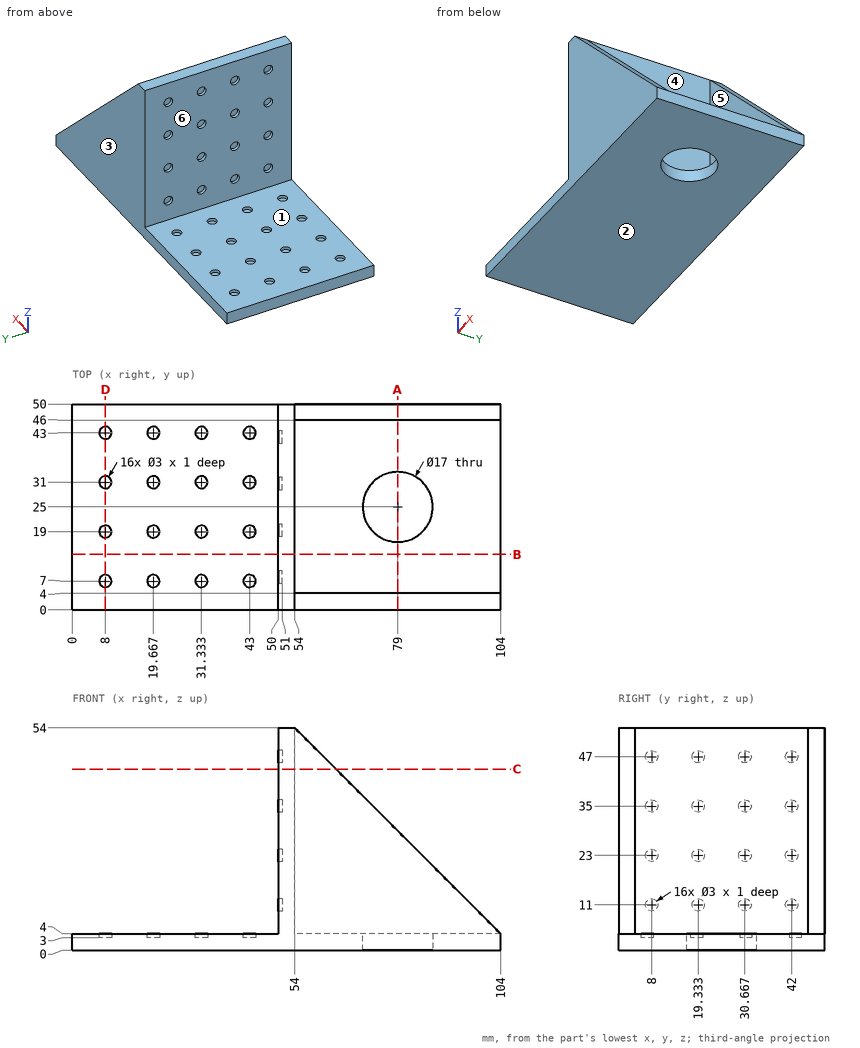
Verification items for this drawing (mm, ordinates from the low corner). A direction names the side the tool comes from. Give positions to 0.01 mm unless a question says otherwise; leave off trailing zeros. Loops run counter-clockwise (first coordinate to the right, second up) from the corner with the lowest first, then second, coordinate; pieces in that order, holes last. Notation, with made-up numbers: M 12,-6.5 L 48,-6.5 A34 ccw 48,29.5 Z; hole C -19.75,16 d4. An arc over 180 degrees is marked long. Answer as a JSON object with one key per item and string values. Group by question number.
Item 1: Sectioned sample at C-C on z = 44. Record the boundary of the cut face in (x, y), plus the area to 3 significant figures.
Item 2: Sectioned sample at D-D on x = 8. Record the boundary of the cut face in (y, z), plus the area to 3 significant figures.
Item 3: Gauge pin test, flat ends, axial feed: pin 1 (3.5 mm diameter, centred on y = 19.33, z = 47, fed in from +X); pin 2 (12 mm diameter, centred on y = 24, z = 23, fed in from -X); pin 3 (4 mm diameter, centred on x = 32.5, y = 28.5, fed in from +Z). Record the tip position at first contact, or that the pin passes through.
Item 4: Access from +Z, -Z, +X, -X, +Y, -Y to the whole of each face (thin tool, end or side, straight path). Record for the marked faces 1 and 2.
Item 5: Sectioned sample at B-B on y = 13.5. Record the boundary of the cut face in (x, z), plus the area to 3 significant figures.
Item 6: Material ranges on L1, parallel to Y at x = 59, z = 39; L2, parallel to Z at x = 34.5, y = 30; L3, parallel to X at y = 28, z = 33, recorded low to high.
Item 7: Mould release check, pull along Y, two halves, no side actions. Record for the marked faces 3, 4, 5 and 6: pulls with the +Y half, pulls with the -Y half, needs draft (parallel to the pull), parting line crosses it, or undercut.
Item 8: Sectioned sample at A-A on x = 79. Record the boundary of the cut face in (y, z), plus the area to 3 significant figures.
Findings below:
{
 "1": {"outline": "M 50,0 L 64,0 L 64,4 L 54,4 L 54,46 L 64,46 L 64,50 L 50,50 Z", "area": "280 mm2"},
 "2": {"outline": "M 0,0 L 50,0 L 50,4 L 44.5,4 L 44.5,3 L 41.5,3 L 41.5,4 L 32.5,4 L 32.5,3 L 29.5,3 L 29.5,4 L 20.5,4 L 20.5,3 L 17.5,3 L 17.5,4 L 8.5,4 L 8.5,3 L 5.5,3 L 5.5,4 L 0,4 Z", "area": "188 mm2"},
 "3": {"pin 1": "x = 54", "pin 2": "x = 50", "pin 3": "z = 4"},
 "4": {"face 1": "+Z, -X, +Y, -Y", "face 2": "-Z, +X, -X, +Y, -Y"},
 "5": {"outline": "M 0,0 L 104,0 L 104,4 L 54,4 L 54,54 L 50,54 L 50,4 L 0,4 Z", "area": "616 mm2"},
 "6": {"L1": "0 to 4, 46 to 50", "L2": "0 to 4", "L3": "50 to 54"},
 "7": {"face 3": "pulls with the +Y half", "face 4": "undercut", "face 5": "undercut", "face 6": "needs draft"},
 "8": {"outline": "M 0,0 L 16.5,0 L 16.5,4 L 4,4 L 4,29 L 0,29 Z; M 33.5,0 L 50,0 L 50,29 L 46,29 L 46,4 L 33.5,4 Z", "area": "332 mm2"}
}
